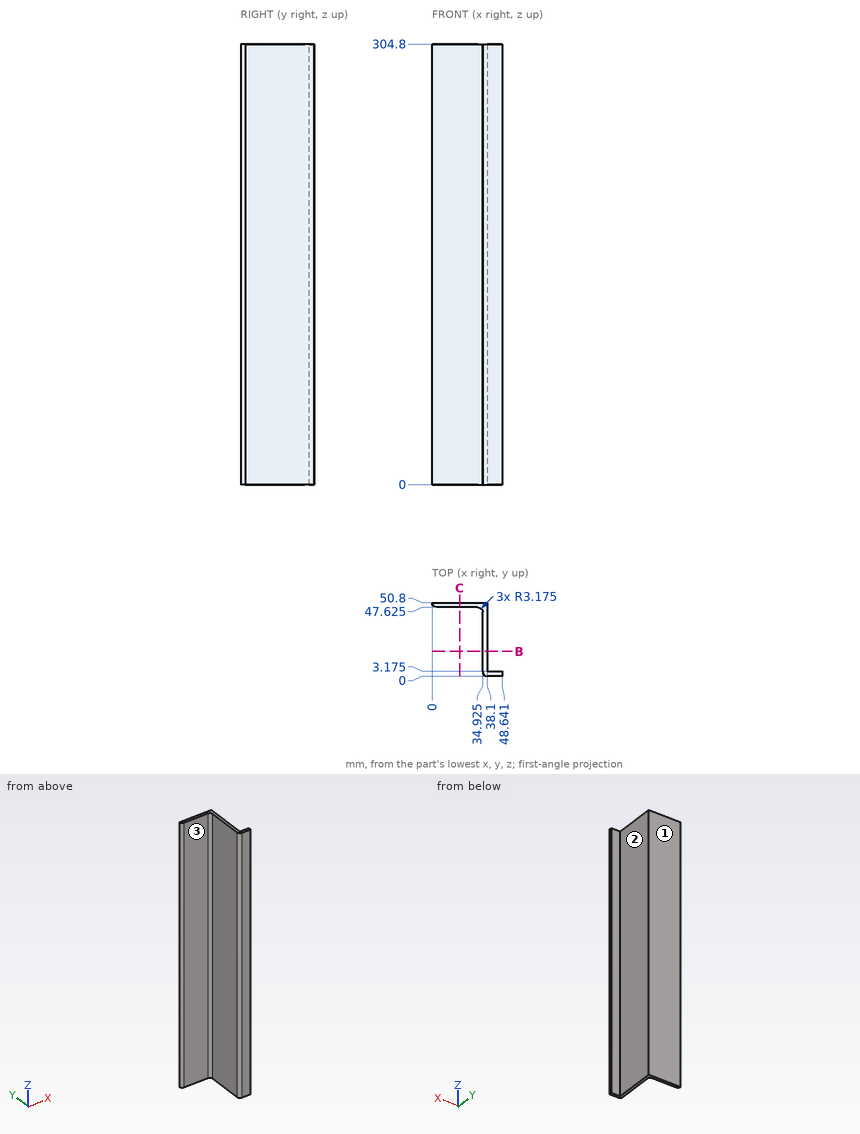
Geometry: see drawing. Coordinates: mm, zero at the bounding-box minimum. A direction names the side the tool comes from. Give positions to 0.01 mm unless a question says otherwise; leave off trailing zeros. Loops run counter-clockwise (first coordinate to the right, second up) from the corner with the lowest first, then second, coordinate; pieces in that order, holes last. Notation, with made-up numbers: (66.25, -36.75) - (122.25, -36.75) arc R16 ccw to (122.25, -9.75) - close; hole circle Ø5 at (0, -31.5). An arc over 180 degrees is marked (long way). Answer as CSV lines item,"result". Start each with the question number.
1. Section C-C, the plane x = 19. Return loops of the section in (y, z) (3 decimals).
2. Reachability of the marked faces 1, 2 and 3 from +Z, -Z, +X, -X, +Y, -Y: full face, straight path, thin tool, end or side. Return the list, or none.
3. Ray query, L1, parallel to X at y = 25.5, z = 171 (3 decimals); L2, parallel to Y at x = 46.5, z = 16.5 (3 decimals); L3, parallel to Y at x = 5, z = 112 (3 decimals). Return the intervals inside material, ascending.
4. Pin query (flat end, axial travel): P1, Ø5, axis at y = 43, z = 265, coming from the +X side; P2, Ø8, axis at x = 12.5, z = 139, coming from the -Y side (3 decimals); P3, Ø5, axis at y = 11, z = 85.5, coming from the -X side (3 decimals). Return the tip coordinate at first contact, or that it passes through.
5. Section B-B, the plane y = 17. Return loops of the section in (x, z) (3 decimals), plus the area to 3 significant figures.
Answers:
1,outline,"(47.625, 0) - (50.8, 0) - (50.8, 304.8) - (47.625, 304.8) - close"
2,face 1,"+Z, -Z, +X, -X, +Y"
2,face 2,"+Z, -Z, +X, +Y"
2,face 3,"+Z, -Z, -X, -Y"
3,L1,"x = 34.925 to 38.1"
3,L2,"y = 0 to 3.175"
3,L3,"y = 47.625 to 50.8"
4,P1,"stops at x = 38.1"
4,P2,"stops at y = 47.625"
4,P3,"stops at x = 34.925"
5,outline,"(34.925, 0) - (38.1, 0) - (38.1, 304.8) - (34.925, 304.8) - close"
5,area,"968 mm2"
